Autodesk Inventor part; units mm, degrees
ref_plane "YZ Plane" through (0, 0, 0) normal (1, 0, 0) x (0, 1, 0)
ref_plane "XZ Plane" through (0, 0, 0) normal (0, 1, 0) x (-1, 0, 0)
ref_plane "XY Plane" through (0, 0, 0) normal (0, 0, 1) x (1, 0, 0)
sketch "Náčrt2" plane through (0, 0, 0) normal (0, 1, 0) x (-1, 0, 0)
  line L0 (67.5, 23.75) -> (-67.5, 23.75)
  line L1 (-67.5, 23.75) -> (-67.5, -23.75)
  line L2 (-67.5, -23.75) -> (67.5, -23.75)
  line L3 (67.5, -23.75) -> (67.5, 23.75)
  point P0 (0, 0)
  point P1 (67.5, 0)
  point P2 (0, 23.75)
  dimension "d0" = 135
  dimension "d1" = 47.5
extrude "Vysunutí1" add sketch "Náčrt2" along normal blind 6
sketch "Náčrt3" plane through (61.5, 6, 23.75) normal (1, 0, 0) x (0, 1, 0)
  line L0 (0, -47.5) -> (0, 0)
  line L1 (0, 0) -> (-70, 0)
  line L2 (-70, 0) -> (-70, -47.5)
  line L3 (-70, -47.5) -> (0, -47.5)
edge flange "Obruba1" height 70 angle 90 thickness 6 bend radius 6 thickness toward (1, 0, 0) relief tear relief width 6 relief depth 3 corner gap 6 corner form 0 edges at (67.5, 0, 0) (-67.5, 0, 0) wall of the first edge with corners at (61.5, 6, -23.75) (61.5, 6, 23.75) (61.5, -64, 23.75) (61.5, -64, -23.75)
bend "Ohyb1"
corner "Roh1"
sketch "Náčrt4" plane through (-67.5, -64, -23.75) normal (0, -1, 0) x (1, 0, 0)
  line L0 (0, 47.5) -> (0, 0) construction
  line L1 (6, 0) -> (0, 0) construction
  line L2 (6, 47.5) -> (6, 0) construction
  line L3 (6, 47.5) -> (0, 47.5) construction
  line L4 (135, 0) -> (135, 47.5) construction
  line L5 (129, 47.5) -> (135, 47.5) construction
  line L6 (129, 0) -> (129, 47.5) construction
  line L7 (129, 0) -> (135, 0) construction
  line L8 (0, 47.5) -> (0, 0)
  line L9 (0, 47.5) -> (6, 47.5)
  line L10 (6, 47.5) -> (6, 37.5)
  line L11 (6, 37.5) -> (0, 37.5)
  line L12 (0, 37.5) -> (0, 47.5)
  line L13 (135, 47.5) -> (129, 47.5)
  line L14 (129, 47.5) -> (129, 37.5)
  line L15 (129, 37.5) -> (135, 37.5)
  line L16 (135, 37.5) -> (135, 47.5)
  point P0 (67.5, 23.75)
  dimension "d18" = 10
extrude "Vysunutí2" add sketch "Náčrt4" along normal blind 31.5
fillet "Zaoblení2" radius 6 4 edges at (64.5, -64, 13.75) (-64.5, -64, 13.75) (-64.5, -95.5, 23.75) (64.5, -95.5, 23.75)
equation "\"d4\" = ŠířkaVýštipu"
equation "\"d5\" = HloubkaVýštipu"
equation "\"d6\" = MinimálníZbytek"
equation "\"d7\" = PoloměrOhybu"
equation "\"d10\" = PoloměrOhybu"
equation "\"d11\" = VelikostRohovéhoVýštipu"
equation "\"d12\" = VelikostMezery"
equation "\"d13\" = VelikostJacobihoPoloměru"
equation "\"PoloměrOhybu\" = Tloušťka"
equation "\"ŠířkaVýštipu\" = Tloušťka"
equation "\"HloubkaVýštipu\" = 0.5 * Tloušťka"
equation "\"VelikostRohovéhoVýštipu\" = 4 * Tloušťka"
equation "\"MinimálníZbytek\" = 2 * Tloušťka"
equation "\"PřechodovýPoloměr\" = PoloměrOhybu"
equation "\"VelikostJacobihoPoloměru\" = PoloměrOhybu"
equation "\"VelikostMezery\" = Tloušťka"
properties part number "DD_KVD_002_05" material "Nerezová ocel"
Model file for the job. Use its own axes, mm. A direction names the side the tool comes from. Give positions to 0.01 mm unless a question says otherwise; leave off trailing zeros. Loops run counter-clockwise (first coordinate to the right, second up) from the corner with the lowest first, then second, coordinate; pieces in that order, holes last. Notation, with made-up numbers: (-16, 42) -> (4, 42) arc R25 ccw to (4, 62) -> close; hole circle Ø11 at (63, -4.5). An arc over 180 degrees is marked (long way). Use a Markdown table: item, result. Add a question column.
(1) Slice it at D-D on y = -2. List the corners of the cut face in (x, z).
(2) Slice it at C-C on x = -5. List the corners of the cut face in (y, z), and give its area (3 significant figures).
(3) Tool access for faces 1 (the flat face through (-61.5, -40, 0)), 2 (the flat face through (64, -64, -8)), 3 (the flat face through (-65, -95.5, 16)): list every direction of +Z, -Z, +X, -X, +Y, -Y with a clear straight run to the whole face (end or side of a thin tool).
(4) Drop flat-ended pins along their axis: pin 1 Ø14 at (y, z) = (-71.5, 1.5) entering from +X; pin 2 Ø5 at (x, y) = (-65, -86.5) entering from -Z; pin 3 Ø1.5 at (x, z) = (9, -9.5) entering from -Y; pin 4 Ø1.8 at (x, z) = (65, -7) entering from -Y. Give the stop position or say it passes through.
(5) Wall check: line 1 along X through (y, z) = (-85, 14.5); line 2 along Y through (x, z) = (34.5, -9.5); line 3 along Y through (x, z) = (-60.5, 20.5). Give the ranges that are in metal, low to high.
(6) Slice it at B-B on z = -4.5. List the corners of the cut face in (x, y).
(7) Slice it at A-A on y = -61. List the corners of the cut face in (x, z), and give its area (3 significant figures).
Filled sheet:
| question | item | result |
|---|---|---|
| 1 | outline | (-66.81, -23.75) -> (-59.97, -23.75) -> (-59.97, 23.75) -> (-66.81, 23.75) -> close; (59.97, -23.75) -> (66.81, -23.75) -> (66.81, 23.75) -> (59.97, 23.75) -> close |
| 2 | outline | (0, -23.75) -> (6, -23.75) -> (6, 23.75) -> (0, 23.75) -> close |
| 2 | area | 285 mm2 |
| 3 | face 1 | +Z, -Z, -Y |
| 3 | face 2 | -Z, +X, -X, -Y |
| 3 | face 3 | +Z, -Z, +X, -X, -Y |
| 4 | pin 1 | through |
| 4 | pin 2 | z = 13.75 |
| 4 | pin 3 | y = 0 |
| 4 | pin 4 | y = -64 |
| 5 | line 1 | -67.5 to -61.5, 61.5 to 67.5 |
| 5 | line 2 | 0 to 6 |
| 5 | line 3 | -2.68 to 4.91 |
| 6 | outline | (-67.5, -64) -> (-61.5, -64) -> (-61.5, -6) arc R6 cw to (-55.5, 0) -> (55.5, 0) arc R6 cw to (61.5, -6) -> (61.5, -64) -> (67.5, -64) -> (67.5, -6) arc R12 ccw to (55.5, 6) -> (-55.5, 6) arc R12 ccw to (-67.5, -6) -> close |
| 7 | outline | (-67.5, -23.75) -> (-61.5, -23.75) -> (-61.5, 23.75) -> (-67.5, 23.75) -> close; (61.5, -23.75) -> (67.5, -23.75) -> (67.5, 23.75) -> (61.5, 23.75) -> close |
| 7 | area | 570 mm2 |
